Read the model definition and answer for the solid it produces. Units are mm, in the model's axes. A direction names the side the tool comes from. Give positions to 0.01 mm unless a question says otherwise; leave off trailing zeros. Order: outer loops, then holes, each group sorted by start corner. A loop starts at its lowest first (then second) coordinate and runs counter-clockwise, first axis right, second up. Notation, with made-up numbers: (27.25, -1) - (80.25, -1) arc R10 ccw to (80.25, 4) - close; hole circle Ø2 at (-7, -3.5). An arc over 180 degrees is marked (long way). Write item = value, one per line.
```python
from build123d import *

# Parameters (mm, degrees)
F1_DEPTH = 200
F2_R     = 5
F3_R     = 10


with BuildPart() as f1:
    # F0 (on Front) → F1 (new body)
    with BuildSketch(Plane.XZ):
        Polygon((100, 0), (0, 0), (0, 50), (-5, 50), (-5, -5), (105, -5), (105, 50), (100, 50), align=None)
    extrude(amount=-F1_DEPTH)

    # F2
    f2_edges = [f1.edges().sort_by_distance(p)[0] for p in [
        (0, 100, 0),
        (100, 100, 0),
    ]]
    fillet(f2_edges, radius=F2_R)

    # F3
    f3_edges = [f1.edges().sort_by_distance(p)[0] for p in [
        (105, 100, -5),
        (-5, 100, -5),
    ]]
    fillet(f3_edges, radius=F3_R)


solid = f1.part
```
1. Determine the mould class of faces 1 (the face through (102.15, 101.4, -1.99)), 2 (the face through (98, 101, 1)), 3 (the face through (50, 200, -2)) for opening direction X: +X half, -X half, draft (parallel to the pull), parting line (faces both ways), or undercut.
Recorded:
face_1 = +X half
face_2 = undercut
face_3 = draft
2. Straight lines are drawn through the part: L1, parallel to X at y = 90, z = 4.5; L2, parallel to Z at x = 56.5, y = 189.5; L3, parallel to X at y = 106, z = 1.5. For each, find the intervals that lie inside material, in ascending order. Write a range as [from, to].
Recorded:
L1 = [-4.99, 0.03], [99.97, 104.99]
L2 = [-5, 0]
L3 = [-4.37, 1.43], [98.57, 104.37]
3. Section A-A (z = 46.5) is taken. Determine the outline of the cut face in (x, y).
Recorded:
outline = (-5, 0) - (0, 0) - (0, 200) - (-5, 200) - close; (100, 0) - (105, 0) - (105, 200) - (100, 200) - close
4. Section B-B (y = 102.5) is taken. Determine the outline of the cut face in (x, z).
Recorded:
outline = (-5, 5) arc R10 ccw to (5, -5) - (95, -5) arc R10 ccw to (105, 5) - (105, 50) - (100, 50) - (100, 5) arc R5 cw to (95, 0) - (5, 0) arc R5 cw to (0, 5) - (0, 50) - (-5, 50) - close
5. Section C-C (x = 88) is taken. Determine the outline of the cut face in (y, z).
Recorded:
outline = (0, -5) - (200, -5) - (200, 0) - (0, 0) - close
6. A flat-ended cylindrical pin translates along its axis: pin 1 (6 mm diameter, centred on x = 85.5, y = 33.5, fed in from +Z). Find the tip coordinate at first contact, or state that the pin passes through.
Recorded:
pin_1 = 0
7. Section D-D (x = 2.5) is taken. Determine the outline of the cut face in (y, z).
Recorded:
outline = (0, -4.68) - (200, -4.68) - (200, 0.67) - (0, 0.67) - close
8. For faces 4 (the face through (50, 0, -2)), 5 (the face through (100, 99, 28)), determine the directions among +Z, -Z, +X, -X, +Y, -Y from which every point of the face is accessible in a straight line to the end or side of a thin tool.
Recorded:
face_4 = +Z, -Z, +X, -X, -Y
face_5 = +Z, +Y, -Y
